For this review, take the finished solid that the model builds, in its own axes (mm). Coordinates: 2 decimals unless noted, no trailing zeros. Loops run counter-clockwise (first coordinate to the right, second up) from the corner with the lowest first, then second, coordinate; pieces in that order, holes last. Notation, with made-up numbers: M 67.25,37.5 L 87.25,37.5 A33 cw 87.25,71.5 Z; hole C 5,82 d1. An arc over 180 degrees is marked long. Answer as a JSON object with one key per item and string values. Group by question number.
Item 1: Wall thickness on L1, parallel to Z at x = 12.7, y = 1.95; L2, parallel to X at y = 23.25, z = -38.1; L3, parallel to Y at x = 20, z = -222 (3 decimals): over which ranges is each line inside the solid? List them lowest first. Write a range as from..to.
Item 2: Add section A-A (z = -295). State the section outline as (x, y) points (3 decimals).
Item 3: Insertion check: pin 1 (3 mm diameter, centred on x = 12.7, z = -577.85, fed in from +Y). The pin has a flat end and moves straight along its axis. Give the tip position at first contact, or say it passes through.
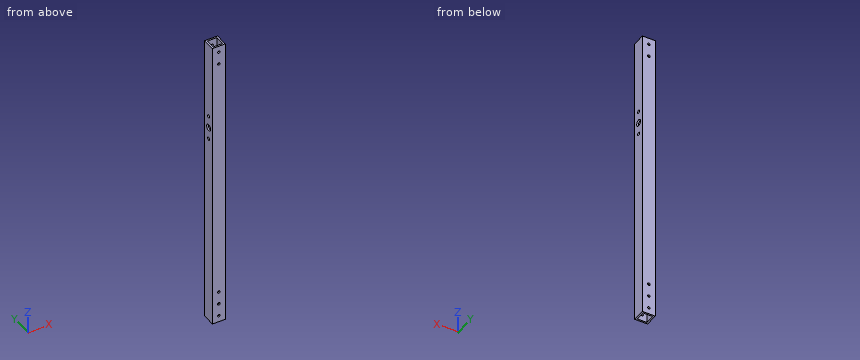
Autodesk Inventor part; units mm, degrees
ref_plane "YZ Plane" through (0, 0, 0) normal (1, 0, 0) x (0, 1, 0)
ref_plane "XZ Plane" through (0, 0, 0) normal (0, 1, 0) x (-1, 0, 0)
ref_plane "XY Plane" through (0, 0, 0) normal (0, 0, 1) x (1, 0, 0)
sketch "Sketch1" plane through (0, 0, 0) normal (0, 0, 1) x (1, 0, 0)
  line L0 (0, 0) -> (25.4, 0)
  line L1 (25.4, 0) -> (25.4, 25.4)
  line L2 (25.4, 25.4) -> (0, 25.4)
  line L3 (0, 25.4) -> (0, 0)
  line L4 (3.175, 22.225) -> (22.225, 22.225)
  line L5 (22.225, 22.225) -> (22.225, 3.175)
  line L6 (22.225, 3.175) -> (3.175, 3.175)
  line L7 (3.175, 3.175) -> (3.175, 22.225)
  dimension "d0" = 25.4
  dimension "d1" = 25.4
  dimension "d2" = 3.175
extrude "Extrusion1" add sketch "Sketch1" against normal blind 590.55
sketch "Sketch4" plane through (0, 25.4, 0) normal (0, 1, 0) x (1, 0, 0)
  line L0 (25.4, 590.55) -> (0, 590.55)
  line L1 (25.4, 0) -> (0, 0)
  point P0 (12.7, 12.7)
  point P1 (12.7, 38.1)
  point P2 (12.7, 577.85)
  point P3 (12.7, 552.45)
  point P4 (12.7, 527.05)
  dimension "d32" = 12.7
  dimension "d33" = 25.4
  dimension "d34" = 12.7
  dimension "d35" = 25.4
  dimension "d36" = 25.4
hole "Hole4" at (12.7, 25.4, -12.7) at (12.7, 25.4, -38.1) at (12.7, 25.4, -577.85) at (12.7, 25.4, -552.45) at (12.7, 25.4, -527.05) direction (0, -1, 0) diameter 5.08 depth 25.4 tip angle 118
sketch "Sketch5" plane through (25.4, 0, 0) normal (1, 0, 0) x (0, 0, -1)
  line L0 (0, 0) -> (0, 25.4)
  point P0 (177.8, 12.7)
  point P1 (153.9875, 12.7)
  point P2 (201.6125, 12.7)
  point P3 (0, 12.7)
  dimension "d44" = 23.8125
  dimension "d45" = 23.8125
  dimension "d46" = 177.8
hole "Hole5" at (25.4, 12.7, -153.9875) at (25.4, 12.7, -201.6125) direction (-1, 0, 0) diameter 6.35 depth 25.4 tip angle 118
hole "Hole6" at (25.4, 12.7, -177.8) direction (-1, 0, 0) diameter 12.7 depth 25.4 tip angle 118
properties part number "new vertical kicker thing"
From the geometry:
{
 "1": {"L1": "z = -590.55..-580.39, -575.31..-554.99, -549.91..-529.59, -524.51..-40.64, -35.56..-15.24, -10.16..0", "L2": "x = 0..10.16, 15.24..25.4", "L3": "y = 0..3.175, 22.225..25.4"},
 "2": {"outline": "M 0,0 L 25.4,0 L 25.4,25.4 L 0,25.4 Z; hole M 3.175,3.175 L 22.225,3.175 L 22.225,22.225 L 3.175,22.225 Z"},
 "3": {"pin 1": "passes through"}
}
